from build123d import *

# Parameters (mm, degrees)
F0_R     = 70
F1_DEPTH = 80
F2_R     = 50
F3_DEPTH = 100
F4_R     = 60
F4_R_2   = 50
F5_DEPTH = 3


with BuildPart() as f1:
    # F0 (on Top) → F1 (new body)
    with BuildSketch(Plane.XY):
        with Locations((-43.891169, -16.593579)):
            Circle(F0_R)
    extrude(amount=F1_DEPTH)

    # F2 (on face) → F3 (cut)
    with BuildSketch(Plane.XY.offset(80)):
        with Locations((-43.891169, -16.593579)):
            Circle(F2_R)
    extrude(amount=-F3_DEPTH, mode=Mode.SUBTRACT)

    # F4 (on face) → F5 (join)
    with BuildSketch(Plane.XY.offset(80)):
        with Locations((-43.891169, -16.593579)):
            Circle(F4_R)
        with Locations((-43.891169, -16.593579)):
            Circle(F4_R_2, mode=Mode.SUBTRACT)
    extrude(amount=F5_DEPTH)


solid = f1.part
Build history of the part. All positions in model axes, mm. A direction names the side the tool comes from. Round coordinates to 2 decimals unless told otherwise and drop trailing zeros. Write each loop counter-clockwise with the first axis right and the second up, starting at its lowest first coordinate (ties: lowest second). Pieces come first, ordered by that corner, then holes. Notation, with made-up numbers: M 48.5,33.5 L 95.5,33.5 A18 ccw 95.5,41.5 Z; hole C 69.5,13 d10. An arc over 180 degrees is marked long. Answer as a JSON object with one key per item and string values. Group by question number.
(1) Flat gauge pins, fed straight in: pin 1 (6 mm diameter, centred on x = -47, z = 13.5, fed in from -Y); pin 2 (10 mm diameter, centred on x = -95.5, y = 29, fed in from +Z); pin 3 (12 mm diameter, centred on x = -93.5, z = 16, fed in from +Y). Where does each tip first touch, or does it go through?
(2) Cut at D-D (z = 15). Give the cut face in (x, y), and give its area (3 significant figures).
(3) Cut at A-A (y = 15). Give the cut face in (x, z).
(4) Which spindle directions (+Z, -Z, +X, -X, +Y, -Y) get a long thin tool onto all of the face, cutting with end or side? Do faces 1 (the flat face through (-58, 33, 83)), 2 (the cylindrical face through (-103.833, -13.955, 81.479)). Say none if no direction does.
(5) Drill centre lines: L1, parallel to X at y = -16.5, z = 63; L2, parallel to Y at x = -59, z = 4; L3, parallel to X at y = -12, z = 68. Where is each one in solid material? Low to high.
(6) Cut at B-B (x = -29). Give the cut face in (y, z).
(7) Cut at C-C (y = -72.5). Give the cut face in (x, z).
Responses:
{
 "1": {"pin 1": "stops at y = -86.59", "pin 2": "stops at z = 80", "pin 3": "stops at y = 38.16"},
 "2": {"outline": "C -43.89,-16.59 d140; hole C -43.89,-16.59 d100", "area": "7,540 mm2"},
 "3": {"outline": "M -106.36,0 L -82.64,0 L -82.64,83 L -94.9,83 L -94.9,80 L -106.36,80 Z; M -5.14,0 L 18.57,0 L 18.57,80 L 7.12,80 L 7.12,83 L -5.14,83 Z"},
 "4": {"face 1": "+Z, +X, -X, +Y, -Y", "face 2": "+Z"},
 "5": {"L1": "x = -113.89 to -93.89, 6.11 to 26.11", "L2": "y = -84.94 to -64.26, 31.07 to 51.76", "L3": "x = -113.74 to -93.68, 5.9 to 25.96"},
 "6": {"outline": "M -84.99,0 L -64.32,0 L -64.32,83 L -74.72,83 L -74.72,80 L -84.99,80 Z; M 31.14,0 L 51.8,0 L 51.8,80 L 41.53,80 L 41.53,83 L 31.14,83 Z"},
 "7": {"outline": "M -86.02,0 L -1.77,0 L -1.77,80 L -22.11,80 L -22.11,83 L -65.67,83 L -65.67,80 L -86.02,80 Z"}
}
